```python
from build123d import *

# Parameters (mm, degrees)
ESQUISSE1_W             = 208
ESQUISSE1_H             = 300
BOSS_EXTRU_1_DEPTH      = 3
ESQUISSE2_W             = 8
ESQUISSE2_H             = 3
ENL_V_MAT_EXTRU_1_DEPTH = 3


with BuildPart() as part:
    # Esquisse1 → Boss.-Extru.1 (new body)
    with BuildSketch(Plane.XY):
        Rectangle(ESQUISSE1_W, ESQUISSE1_H)
    extrude(amount=BOSS_EXTRU_1_DEPTH)

    # Esquisse2 → Enlèv. mat.-Extru.1 (cut)
    with BuildSketch(Plane.XY.offset(3)):
        with Locations((-92, 148.5)):
            Rectangle(ESQUISSE2_W, ESQUISSE2_H)
        with Locations((-76, 148.5)):
            Rectangle(ESQUISSE2_W, ESQUISSE2_H)
        with Locations((-60, 148.5)):
            Rectangle(ESQUISSE2_W, ESQUISSE2_H)
        with Locations((-44, 148.5)):
            Rectangle(ESQUISSE2_W, ESQUISSE2_H)
        with Locations((-28, 148.5)):
            Rectangle(ESQUISSE2_W, ESQUISSE2_H)
        with Locations((-12, 148.5)):
            Rectangle(ESQUISSE2_W, ESQUISSE2_H)
        with Locations((4, 148.5)):
            Rectangle(ESQUISSE2_W, ESQUISSE2_H)
        with Locations((20, 148.5)):
            Rectangle(ESQUISSE2_W, ESQUISSE2_H)
        with Locations((36, 148.5)):
            Rectangle(ESQUISSE2_W, ESQUISSE2_H)
        with Locations((52, 148.5)):
            Rectangle(ESQUISSE2_W, ESQUISSE2_H)
        with Locations((68, 148.5)):
            Rectangle(ESQUISSE2_W, ESQUISSE2_H)
        with Locations((84, 148.5)):
            Rectangle(ESQUISSE2_W, ESQUISSE2_H)
        with Locations((100, 148.5)):
            Rectangle(ESQUISSE2_W, ESQUISSE2_H)
        with Locations((100, -148.5)):
            Rectangle(ESQUISSE2_W, ESQUISSE2_H)
        with Locations((84, -148.5)):
            Rectangle(ESQUISSE2_W, ESQUISSE2_H)
        with Locations((68, -148.5)):
            Rectangle(ESQUISSE2_W, ESQUISSE2_H)
        with Locations((52, -148.5)):
            Rectangle(ESQUISSE2_W, ESQUISSE2_H)
        with Locations((36, -148.5)):
            Rectangle(ESQUISSE2_W, ESQUISSE2_H)
        with Locations((20, -148.5)):
            Rectangle(ESQUISSE2_W, ESQUISSE2_H)
        with Locations((4, -148.5)):
            Rectangle(ESQUISSE2_W, ESQUISSE2_H)
        with Locations((-12, -148.5)):
            Rectangle(ESQUISSE2_W, ESQUISSE2_H)
        with Locations((-28, -148.5)):
            Rectangle(ESQUISSE2_W, ESQUISSE2_H)
        with Locations((-44, -148.5)):
            Rectangle(ESQUISSE2_W, ESQUISSE2_H)
        with Locations((-60, -148.5)):
            Rectangle(ESQUISSE2_W, ESQUISSE2_H)
        with Locations((-76, -148.5)):
            Rectangle(ESQUISSE2_W, ESQUISSE2_H)
        with Locations((-92, -148.5)):
            Rectangle(ESQUISSE2_W, ESQUISSE2_H)
    extrude(amount=-ENL_V_MAT_EXTRU_1_DEPTH, mode=Mode.SUBTRACT)


solid = part.part
```
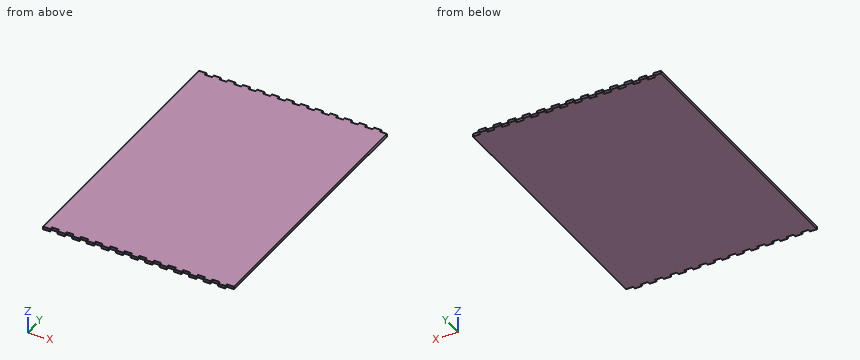
CAD build for the part. Positions are in the model's coordinates, mm. Give positions to 0.01 mm unless a question says otherwise; leave off trailing zeros. Write each loop counter-clockwise with the first axis right and the second up, starting at its lowest first coordinate (ties: lowest second). Pieces come first, ordered by that corner, then holes. Notation, with made-up numbers: M 40.25,-38.5 L 81.25,-38.5 A25 cw 81.25,-1.5 Z; hole C 24,63.25 d7. An arc over 180 degrees is marked long. Return JSON: item names as keys, results as strings. Group by question number.
(1) Flat gauge pins, fed straight in: pin 1 Ø1.5 at (x, z) = (37.5, 2) entering from +Y; pin 2 Ø1.5 at (x, z) = (-76, 1.5) entering from -Y; pin 3 Ø1.5 at (y, z) = (149, 1.5) entering from +X. Where does each tip first touch, or does it go through?
(2) Band-saw the part on A-A (x = 51.5). Give the cut face in (y, z).
(3) Drill centre line: L1, parallel to Y at x = 3.5, z = 0.25. Where is it in solid material? Low to high. Write a range as [from, to].
Entries:
{
 "1": {"pin 1": "stops at y = 147", "pin 2": "stops at y = -147", "pin 3": "stops at x = 96"},
 "2": {"outline": "M -147,0 L 147,0 L 147,3 L -147,3 Z"},
 "3": {"L1": "y = [-147, 147]"}
}
